Verification items for the finished model (mm, model axes). A direction names the side the tool comes from. Round coordinates to 2 decimals unless told otherwise and drop trailing zeros. Write each loop counter-clockwise with the first axis right and the second up, starting at its lowest first coordinate (ties: lowest second). Pieces come first, ordered by that corner, then holes.
from build123d import *

# Parameters (mm, degrees)
BOSS_EXTRUDE1_DEPTH = 100
SKETCH2_R           = 10
CUT_EXTRUDE1_DEPTH  = 7.5
CUT_EXTRUDE2_DEPTH  = 4.75
SKETCH6_R           = 1
CUT_EXTRUDE3_DEPTH  = 6
SKETCH7_W           = 9.5
SKETCH7_H           = 7.367856256
CUT_EXTRUDE4_DEPTH  = 6
SKETCH8_W           = 9.5
SKETCH8_H           = 7.367856256
BOSS_EXTRUDE2_DEPTH = 12.5
SKETCH10_R          = 10
CUT_EXTRUDE5_DEPTH  = 68
FILLET1_R           = 5
CUT_EXTRUDE6_DEPTH  = 5
SKETCH13_W          = 9.5
SKETCH13_H          = 3
CUT_EXTRUDE7_DEPTH  = 5
CUT_EXTRUDE8_DEPTH  = 12.5
CUT_EXTRUDE9_DEPTH  = 5
SKETCH17_W          = 11
SKETCH17_H          = 9.5
CUT_EXTRUDE11_DEPTH = 90


with BuildPart() as part:
    # Sketch1 → Boss-Extrude1 (new body)
    with BuildSketch(Plane(origin=(0, 0, 0), x_dir=(1, 0, 0), z_dir=(0, 1, 0))):
        with BuildLine():
            Line((-4.0452326, 19.590813971), (5.9547674, 19.590813971))
            Line((5.9547674, 19.590813971), (5.9547674, -0.409186029))
            Line((5.9547674, -0.409186029), (5.9547674, -20.409186029))
            Line((5.9547674, -20.409186029), (-4.0452326, -20.409186029))
            ThreePointArc((-4.0452326, -20.409186029), (-11.116300412, -17.48025384), (-14.0452326, -10.409186029))
            Line((-14.0452326, -10.409186029), (-14.0452326, 9.590813971))
            ThreePointArc((-14.0452326, 9.590813971), (-11.116300412, 16.661881783), (-4.0452326, 19.590813971))
        make_face()
    extrude(amount=BOSS_EXTRUDE1_DEPTH)

    # Sketch2 → Cut-Extrude1 (cut)
    with BuildSketch(Plane(origin=(5.9547674, 0, 0), x_dir=(0, 0, -1), z_dir=(1, 0, 0))):
        with Locations((-0.409186029, 68.83)):
            Circle(SKETCH2_R)
    extrude(amount=-CUT_EXTRUDE1_DEPTH, mode=Mode.SUBTRACT)

    # Sketch4 → Cut-Extrude2 (cut, symmetric)
    with BuildSketch(Plane.XY):
        Polygon((-1.5452326, 89.777572113), (3.4547674, 89.777572113), (3.4547674, 12.777572113), (3.4547674, 5.409715857), (-15.452876316, 5.409715857), (-15.452876316, 12.777572113), (-1.5452326, 12.777572113), align=None)
    extrude(amount=CUT_EXTRUDE2_DEPTH, both=True, mode=Mode.SUBTRACT)

    # Sketch6 → Cut-Extrude3 (cut)
    with BuildSketch(Plane.XZ):
        with Locations((-4.0452326, -9.590813971)):
            Circle(SKETCH6_R)
        with Locations((-4.0452326, 10.409186029)):
            Circle(SKETCH6_R)
    extrude(amount=-CUT_EXTRUDE3_DEPTH, mode=Mode.SUBTRACT)

    # Sketch7 → Cut-Extrude4 (cut)
    with BuildSketch(Plane.ZY.offset(-3.4547674)):
        with Locations((0, 9.093643985)):
            Rectangle(SKETCH7_W, SKETCH7_H)
    extrude(amount=-CUT_EXTRUDE4_DEPTH, mode=Mode.SUBTRACT)

    # Sketch8 → Boss-Extrude2 (add)
    with BuildSketch(Plane.ZY.offset(14.0452326)):
        with Locations((0, 9.093643985)):
            Rectangle(SKETCH8_W, SKETCH8_H)
    extrude(amount=-BOSS_EXTRUDE2_DEPTH)

    # Sketch10 → Cut-Extrude5 (cut)
    with BuildSketch(Plane(origin=(5.9547674, 0, 0), x_dir=(0, 0, -1), z_dir=(1, 0, 0))):
        with Locations((-0.409186029, 68.83)):
            Circle(SKETCH10_R)
    extrude(amount=-CUT_EXTRUDE5_DEPTH, mode=Mode.SUBTRACT)

    # Fillet1
    fillet1_edges = [part.edges().sort_by_distance(p)[0] for p in [
        (-11.116300412, 100, -16.661881783),
        (-14.0452326, 100, 0.409186029),
        (-11.116300412, 100, 17.48025384),
        (0.9547674, 100, 20.409186029),
        (0.9547674, 100, -19.590813971),
    ]]
    fillet(fillet1_edges, radius=FILLET1_R)

    # Sketch11 → Cut-Extrude6 (cut)
    with BuildSketch(Plane(origin=(-1.5452326, 0, 0), x_dir=(0, 0, -1), z_dir=(1, 0, 0))):
        with BuildLine():
            Line((-4.75, 59.821263459), (-4.75, 5.409715857))
            Line((-4.75, 5.409715857), (4.75, 5.409715857))
            Line((4.75, 5.409715857), (4.75, 60.263623898))
            ThreePointArc((4.75, 60.263623898), (0.055952548, 58.840823552), (-4.75, 59.821263459))
        make_face()
    extrude(amount=-CUT_EXTRUDE6_DEPTH, mode=Mode.SUBTRACT)

    # Sketch13 → Cut-Extrude7 (cut)
    with BuildSketch(Plane(origin=(5.9547674, 0, 0), x_dir=(0, 0, -1), z_dir=(1, 0, 0))):
        with Locations((0, 14.277572113)):
            Rectangle(SKETCH13_W, SKETCH13_H)
    extrude(amount=-CUT_EXTRUDE7_DEPTH, mode=Mode.SUBTRACT)

    # Sketch14 → Cut-Extrude8 (cut)
    with BuildSketch(Plane(origin=(5.9547674, 0, 0), x_dir=(0, 0, -1), z_dir=(1, 0, 0))):
        with BuildLine():
            Line((4.75, 15.777572113), (-4.75, 15.777572113))
            ThreePointArc((-4.75, 15.777572113), (0, 18.113561026), (4.75, 15.777572113))
        make_face()
    extrude(amount=-CUT_EXTRUDE8_DEPTH, mode=Mode.SUBTRACT)

    # Sketch16 → Cut-Extrude9 (cut)
    with BuildSketch(Plane(origin=(-1.5452326, 0, 0), x_dir=(0, 0, -1), z_dir=(1, 0, 0))):
        with BuildLine():
            ThreePointArc((-4.75, 89.777572113), (0, 93.055148297), (4.75, 89.777572113))
            Line((4.75, 89.777572113), (-4.75, 89.777572113))
        make_face()
    extrude(amount=CUT_EXTRUDE9_DEPTH, mode=Mode.SUBTRACT)

    # Sketch17 → Cut-Extrude11 (cut)
    with BuildSketch(Plane(origin=(0, 5.409715857, 0), x_dir=(1, 0, 0), z_dir=(0, 1, 0))):
        with BuildLine():
            Line((4.4547674, 4.75), (4.4547674, 18.090813971))
            Line((4.4547674, 18.090813971), (-4.0452326, 18.090813971))
            ThreePointArc((-4.0452326, 18.090813971), (-10.05564024, 15.601221612), (-12.5452326, 9.590813971))
            Line((-12.5452326, 9.590813971), (-12.5452326, -10.409186029))
            ThreePointArc((-12.5452326, -10.409186029), (-10.05564024, -16.419593669), (-4.0452326, -18.909186029))
            Line((-4.0452326, -18.909186029), (4.4547674, -18.909186029))
            Line((4.4547674, -18.909186029), (4.4547674, -4.75))
            Line((4.4547674, -4.75), (-6.5452326, -4.75))
            Line((-6.5452326, -4.75), (-6.5452326, 4.75))
            Line((-6.5452326, 4.75), (4.4547674, 4.75))
        make_face()
        with Locations((-1.0452326, 0)):
            Rectangle(SKETCH17_W, SKETCH17_H)
    extrude(amount=CUT_EXTRUDE11_DEPTH, mode=Mode.SUBTRACT)


solid = part.part
Q1. Release check for a two-part mould opening along Y. For faces 1 (the flat face through (-1, 100, 0)), 2 (the flat face through (0, 50, 18.909)), 3 (the cylindrical face through (5.215, 78.745, 1.711)), 4 (the flat face through (-14.045, 27, 0)) record: released by +Y, released by -Y, zero draft, split by the parting line, or undercut.
Recorded:
face 1: released by +Y
face 2: undercut
face 3: undercut
face 4: zero draft
Q2. Sectioned sample at D-D (z = 7.5). Enter the section's corners in (x, y).
Recorded:
outline: (-14.05, 0) - (5.95, 0) - (5.95, 61.78) - (4.45, 61.78) - (4.45, 5.41) - (-12.55, 5.41) - (-12.55, 61.78) - (-14.05, 61.78) - close; (-14.05, 75.88) - (-12.55, 75.88) - (-12.55, 95.41) - (4.45, 95.41) - (4.45, 75.88) - (5.95, 75.88) - (5.95, 100) - (-9.05, 100) arc R5 ccw to (-14.05, 95) - close
Q3. Tool access check on faces 5 (the flat face through (-4, 95.41, 0)), 6 (the cylindrical face through (-3.584, 2.667, 9.522)), 7 (the cylindrical face through (5.215, 18.113, 0.077)). Record the directions out of +Z, -Z, +X, -X, +Y, -Y that give a thin tool (end or side, any length) a straight path to the whole face; none if there is none.
Recorded:
face 5: none
face 6: -Y
face 7: +X
Q4. Sectioned sample at C-C (z = -3). Enter the section's corners in (x, y).
Recorded:
outline: (-14.05, 0) - (5.95, 0) - (5.95, 5.41) - (-12.55, 5.41) - (-12.55, 59.43) - (-14.05, 59.43) - close; (-14.05, 78.23) - (-12.55, 78.23) - (-12.55, 95.41) - (4.45, 95.41) - (4.45, 78.23) - (5.95, 78.23) - (5.95, 100) - (-9.05, 100) arc R5 ccw to (-14.05, 95) - close; (4.45, 17.31) - (5.95, 17.31) - (5.95, 59.43) - (4.45, 59.43) - close
Q5. Material ranges on line 1 along X through (y, z) = (62.5, -7.5); line 2 along Z through (x, y) = (-2, 80); line 3 along Y through (x, z) = (0.25, -14), recorded low to high.
Recorded:
line 1: x = -14.05 to -12.55, 4.45 to 5.95
line 2: z = -19.59 to -18.09, 18.91 to 20.41
line 3: y = 0 to 5.41, 95.41 to 100
Q6. Sectioned sample at B-B (x = 2.75). Enter the section's corners in (y, z).
Recorded:
outline: (0, -19.59) - (95, -19.59) arc R5 ccw to (100, -14.59) - (100, 15.41) arc R5 ccw to (95, 20.41) - (0, 20.41) - close; hole (5.41, -18.09) - (95.41, -18.09) - (95.41, 18.91) - (5.41, 18.91) - close
Q7. Depth check by flat-ended pin: P1, Ø4, axis at y = 59, z = -1, coming from the -X side; P2, Ø12, axis at y = 68.83, z = 0.41, coming from the -X side; P3, Ø1.2, axis at x = -4.05, z = 10.41, coming from the -Y side; P4, Ø1, axis at x = -10.5, z = -5, coming from the +Y side. Enter the tip coordinate at first touch or a pass-through.
Recorded:
P1: stops at x = -14.05
P2: passes through
P3: stops at y = 95.41
P4: stops at y = 99.91
Q8. Sectioned sample at A-A (y = 56). Enter the section's corners in (x, z).
Recorded:
outline: (-14.05, -9.59) arc R10 ccw to (-4.05, -19.59) - (5.95, -19.59) - (5.95, 20.41) - (-4.05, 20.41) arc R10 ccw to (-14.05, 10.41) - close; hole (-12.55, -9.59) arc R8.5 ccw to (-4.05, -18.09) - (4.45, -18.09) - (4.45, 18.91) - (-4.05, 18.91) arc R8.5 ccw to (-12.55, 10.41) - close
